Model file for the job. Use its own axes, mm. A direction names the side the tool comes from. Round coordinates to 2 decimals unless told otherwise and drop trailing zeros.
```python
from build123d import *

# Parameters (mm, degrees)
PAD_DEPTH           = 6
SKETCH001_W         = 156
SKETCH001_H         = 8.81
POCKET_DEPTH        = 4
SKETCH015_W         = 10
SKETCH015_H         = 10
POCKET001_DEPTH     = 6.001
SKETCH016_W         = 3
SKETCH016_H         = 30
PAD001_DEPTH        = 40
LINEARPATTERN_COUNT = 2
LINEARPATTERN_PITCH = 199
SKETCH017_W         = 196
SKETCH017_H         = 3
PAD002_DEPTH        = 40
SKETCH018_W         = 195.94
SKETCH018_H         = 2
PAD003_DEPTH        = 20


with BuildPart() as part:
    # Sketch → Pad (new body)
    with BuildSketch(Plane.XZ):
        Polygon((-69.143125, 50.802246), (72.856875, 50.802246), (102.86, 50.802246), (102.86, 80.802246), (-99.143366, 80.802246), (-99.143366, 50.802246), align=None)
    extrude(amount=PAD_DEPTH)

    # Sketch001 → Pocket (cut)
    with BuildSketch(Plane(origin=(0, 0, 0), x_dir=(1, 0, 0), z_dir=(0, 1, 0))):
        with Locations((0, -55.095)):
            Rectangle(SKETCH001_W, SKETCH001_H)
    extrude(amount=-POCKET_DEPTH, mode=Mode.SUBTRACT)

    # Sketch015 → Pocket001 (cut, through all)
    with BuildSketch(Plane.XZ.offset(6)):
        with Locations((-46.15, 67.3)):
            Rectangle(SKETCH015_W, SKETCH015_H)
        with Locations((-27.51, 67.3)):
            Rectangle(SKETCH015_W, SKETCH015_H)
        with Locations((-8.87, 67.3)):
            Rectangle(SKETCH015_W, SKETCH015_H)
        with Locations((9.77, 67.3)):
            Rectangle(SKETCH015_W, SKETCH015_H)
        with Locations((28.41, 67.3)):
            Rectangle(SKETCH015_W, SKETCH015_H)
        with Locations((47.05, 67.3)):
            Rectangle(SKETCH015_W, SKETCH015_H)
    extrude(amount=-POCKET001_DEPTH, mode=Mode.SUBTRACT)

    # Sketch016 (on Face4 of Pocket001) → Pad001 (join)
    with BuildSketch(Plane(origin=(0, 0, 0), x_dir=(1, 0, 0), z_dir=(0, 1, 0))):
        with Locations((101.359965, -65.804146)):
            Rectangle(SKETCH016_W, SKETCH016_H)
    pad001 = extrude(amount=PAD001_DEPTH)

    # LinearPattern: Pad001 ×2
    with Locations(*[(-i * LINEARPATTERN_PITCH, 0, 0) for i in range(1, LINEARPATTERN_COUNT)]):
        add(pad001)

    # Sketch017 (on Face4 of LinearPattern) → Pad002 (join)
    with BuildSketch(Plane(origin=(0, 0, 0), x_dir=(1, 0, 0), z_dir=(0, 1, 0))):
        with Locations((1.848167, -79.3)):
            Rectangle(SKETCH017_W, SKETCH017_H)
    extrude(amount=PAD002_DEPTH)

    # Sketch018 (on Face21 of Pad002) → Pad003 (join)
    with BuildSketch(Plane(origin=(0, 0, 77.8), x_dir=(1, 0, 0), z_dir=(0, 0, -1))):
        with Locations((1.86, -10.45)):
            Rectangle(SKETCH018_W, SKETCH018_H)
    extrude(amount=PAD003_DEPTH)


solid = part.part
```
1) Which spindle directions (+Z, -Z, +X, -X, +Y, -Y) get a long thin tool onto all of the face, cutting with end or side? Do faces 4 (the face through (102.86, 20, 66)), 5 (the face through (-46, -3, 62.3)). Say none if no direction does.
2) Flat gauge pins, fed straight in: pin 1 Ø3 at (x, z) = (-37.5, 75.5) entering from +Y; pin 2 Ø5 at (x, y) = (-26.5, -3) entering from -Z; pin 3 Ø12 at (x, y) = (59.5, 10) entering from -Z; pin 4 Ø2 at (x, y) = (-6.5, 2.5) entering from -Z. Where does each tip first touch, or does it go through?
3) Pull direction Y, two halves, no side cores. Call faces 1 (the face through (47, -3, 72.3)), 2 (the face through (0, 20, 77.8)), 3 (the face through (0, -6, 66)): released by +Y, released by -Y, zero draft, split by the parting line, or undercut.
4) Cut at D-D on z = 67.5. Give the number of separate pieces and of enclosed holes in the cut face, and give its area (3 significant figures).
5) Wall check: probe 1 along X at (y, z) = (0.5, 77.5); probe 2 along Y at (x, z) = (-76, 73.5); probe 3 along Z at (x, y) = (33, -1.5). Give the ranges that are in metal, low to high.
Result sheet:
1. face 4: +Z, -Z, +X, +Y, -Y
1. face 5: -Y
2. pin 1: stops at y = 11.45
2. pin 2: stops at z = 50.8
2. pin 3: stops at z = 57.8
2. pin 4: stops at z = 77.8
3. face 1: zero draft
3. face 2: undercut
3. face 3: released by -Y
4. separate pieces: 8
4. enclosed holes: 0
4. area: 1,480 mm2
5. probe 1: x = -99.14 to -96.14, 99.86 to 102.86
5. probe 2: y = -6 to 0, 9.45 to 11.45
5. probe 3: z = 59.5 to 62.3, 72.3 to 80.8
